CAD build for the part. Positions are in the model's coordinates, mm. Face numbers are marked on the shaded views. A direction names the side the tool comes from. Give positions to 0.01 mm unless a question says otherwise; leave off trailing zeros. Order: outer loops, then holes, each group sorted by start corner. A loop starts at its lowest first (then second) coordinate and runs counter-clockwise, first axis right, second up.
```python
from build123d import *

# Parameters (mm, degrees)
SKETCH_W        = 196
SKETCH_H        = 200
PAD_DEPTH       = 3
SKETCH001_R     = 39.5
SKETCH001_R_2   = 2
POCKET_DEPTH    = 5
SKETCH002_W     = 4
SKETCH002_H     = 8
POCKET001_DEPTH = 5
SKETCH003_W     = 8
SKETCH003_H     = 180
PAD001_DEPTH    = 4
SKETCH004_W     = 160
SKETCH004_H     = 8
PAD002_DEPTH    = 4
CHAMFER_SIZE    = 3.99
CHAMFER001_SIZE = 3.99


with BuildPart() as part:
    # Sketch → Pad (new body)
    with BuildSketch(Plane.XY):
        Rectangle(SKETCH_W, SKETCH_H)
    extrude(amount=PAD_DEPTH)

    # Sketch001 (on Face6 of Pad) → Pocket (cut)
    with BuildSketch(Plane.XY.offset(3)):
        with Locations((-50, 50)):
            Circle(SKETCH001_R)
        with Locations((50, 50)):
            Circle(SKETCH001_R)
        with Locations((50, -50)):
            Circle(SKETCH001_R)
        with Locations((-50, -50)):
            Circle(SKETCH001_R)
        with Locations((-85, 85)):
            Circle(SKETCH001_R_2)
        with Locations((-15, 85)):
            Circle(SKETCH001_R_2)
        with Locations((-85, 15)):
            Circle(SKETCH001_R_2)
        with Locations((-15, 15)):
            Circle(SKETCH001_R_2)
        with Locations((15, 15)):
            Circle(SKETCH001_R_2)
        with Locations((15, 85)):
            Circle(SKETCH001_R_2)
        with Locations((85, 85)):
            Circle(SKETCH001_R_2)
        with Locations((85, 15)):
            Circle(SKETCH001_R_2)
        with Locations((85, -15)):
            Circle(SKETCH001_R_2)
        with Locations((15, -15)):
            Circle(SKETCH001_R_2)
        with Locations((15, -85)):
            Circle(SKETCH001_R_2)
        with Locations((85, -85)):
            Circle(SKETCH001_R_2)
        with Locations((-15, -85)):
            Circle(SKETCH001_R_2)
        with Locations((-85, -15)):
            Circle(SKETCH001_R_2)
        with Locations((-15, -15)):
            Circle(SKETCH001_R_2)
        with Locations((-85, -85)):
            Circle(SKETCH001_R_2)
    extrude(amount=-POCKET_DEPTH, mode=Mode.SUBTRACT)

    # Sketch002 (on Face5 of Pocket) → Pocket001 (cut)
    with BuildSketch(Plane.XY.offset(3)):
        with Locations((92, 76)):
            Rectangle(SKETCH002_W, SKETCH002_H)
        with Locations((92, -76)):
            Rectangle(SKETCH002_W, SKETCH002_H)
        with Locations((92, 0)):
            Rectangle(SKETCH002_W, SKETCH002_H)
        with Locations((-92, 0)):
            Rectangle(SKETCH002_W, SKETCH002_H)
        with Locations((-92, 76)):
            Rectangle(SKETCH002_W, SKETCH002_H)
        with Locations((-92, -76)):
            Rectangle(SKETCH002_W, SKETCH002_H)
    extrude(amount=-POCKET001_DEPTH, mode=Mode.SUBTRACT)

    # Sketch003 (on Face5 of Pocket001) → Pad001 (join)
    with BuildSketch(Plane.XY.offset(3)):
        Rectangle(SKETCH003_W, SKETCH003_H)
    extrude(amount=PAD001_DEPTH)

    # Sketch004 (on Face5 of Pad001) → Pad002 (join)
    with BuildSketch(Plane.XY.offset(3)):
        Rectangle(SKETCH004_W, SKETCH004_H)
    extrude(amount=PAD002_DEPTH)

    # Chamfer
    chamfer_edges = [part.edges().sort_by_distance(p)[0] for p in [
        (-42, -4, 7),
        (-42, 4, 7),
        (42, 4, 7),
        (42, -4, 7),
    ]]
    chamfer(chamfer_edges, length=CHAMFER_SIZE)

    # Chamfer001
    chamfer001_edges = [part.edges().sort_by_distance(p)[0] for p in [
        (-4, 47, 7),
        (4, 47, 7),
        (4, -47, 7),
        (-4, -47, 7),
    ]]
    chamfer(chamfer001_edges, length=CHAMFER001_SIZE)


solid = part.part
```
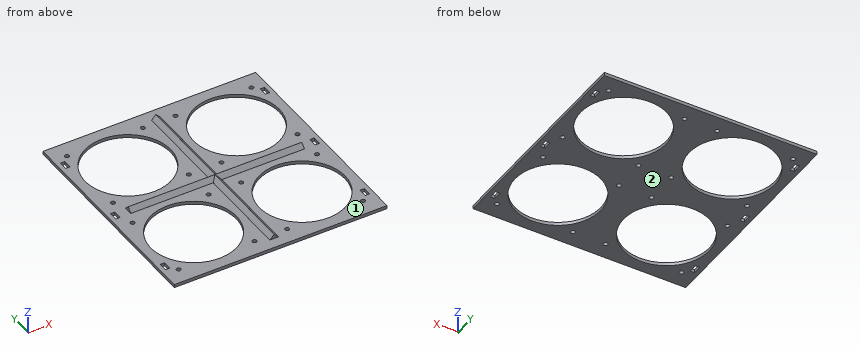
Item 1: Slice it at A-A (x = -50). State how many separate pieces and enclosed holes the cut face has, and give its area (3 significant figures).
Item 2: Slice it at C-C (z = 5). Give the cut face in (x, y).
Item 3: Tool access for the marked faces 1 and 2: list every direction of +Z, -Z, +X, -X, +Y, -Y with a clear straight run to the whole face (end or side of a thin tool).
Item 4: Drop flat-ended pins along their axis: pin 1 Ø4.5 at (x, y) = (85, -85) entering from +Z; pin 2 Ø1 at (x, y) = (-1, 28) entering from +Z. Give the stop position or say it passes through.
Item 5: Wall check: L1, parallel to Y at x = 63.5, z = 2.25; L2, parallel to Y at x = -62.5, z = 0.5; L3, parallel to X at y = 67.5, z = 2.25. Give the ranges that are in metal, low to high.
A:
1. separate pieces: 3
1. enclosed holes: 0
1. area: 142 mm2
2. outline: (-80, -2.01) - (-2.01, -2.01) - (-2.01, -90) - (2.01, -90) - (2.01, -2.01) - (80, -2.01) - (80, 2.01) - (2.01, 2.01) - (2.01, 90) - (-2.01, 90) - (-2.01, 2.01) - (-80, 2.01) - close
3. face 1: +Z
3. face 2: -Z, +X, -X, +Y, -Y
4. pin 1: stops at z = 3
4. pin 2: stops at z = 6.51
5. L1: y = -100 to -87.12, -12.88 to 12.88, 87.12 to 100
5. L2: y = -100 to -87.47, -12.53 to 12.53, 87.47 to 100
5. L3: x = -98 to -85.41, -14.59 to 14.59, 85.41 to 98
